from build123d import *

# Parameters (mm, degrees)
SKETCH1_W               = 20
SKETCH1_H               = 13
SKETCH1_R               = 1.2
BOSS_EXTRUDE1_DEPTH     = 5.8
SKETCH2_R               = 2.5
CUT_EXTRUDE1_DEPTH      = 2
SKETCH3_R               = 1.5
CUT_EXTRUDE2_DEPTH      = 10
FILLET1_R               = 10
FILLET2_R               = 5
FILLET3_R               = 2
FILLET4_R               = 1
SKETCH5_R               = 1.2
BOSS_EXTRUDE2_DEPTH     = 3.9
CUT_EXTRUDE3_DEPTH      = 26.750534103
CUT_EXTRUDE3_DEPTH_BACK = 26.750534103
SKETCH6_R               = 1


with BuildPart() as part:
    # Sketch1 → Boss-Extrude1 (new body)
    with BuildSketch(Plane.XY):
        with Locations((10, 6.5)):
            Rectangle(SKETCH1_W, SKETCH1_H)
        with Locations((16.5, 5)):
            Circle(SKETCH1_R, mode=Mode.SUBTRACT)
    extrude(amount=BOSS_EXTRUDE1_DEPTH)

    # Sketch2 → Cut-Extrude1 (cut)
    with BuildSketch(Plane.XY.offset(5.8)):
        with Locations((16.5, 5)):
            Circle(SKETCH2_R)
    extrude(amount=-CUT_EXTRUDE1_DEPTH, mode=Mode.SUBTRACT)

    # Sketch3 → Cut-Extrude2 (cut)
    with BuildSketch(Plane.ZY):
        with Locations((2.8, 5)):
            Circle(SKETCH3_R)
    extrude(amount=-CUT_EXTRUDE2_DEPTH, mode=Mode.SUBTRACT)

    # Fillet1
    fillet1_edges = [part.edges().sort_by_distance(p)[0] for p in [
        (20, 13, 2.9),
    ]]
    fillet(fillet1_edges, radius=FILLET1_R)

    # Fillet2
    fillet2_edges = [part.edges().sort_by_distance(p)[0] for p in [
        (0, 13, 2.9),
    ]]
    fillet(fillet2_edges, radius=FILLET2_R)

    # Fillet3
    fillet3_edges = [part.edges().sort_by_distance(p)[0] for p in [
        (0, 0, 2.9),
        (20, 0, 2.9),
    ]]
    fillet(fillet3_edges, radius=FILLET3_R)

    # Fillet4
    # the kernel refuses this fillet: 1 mm, written as the material it takes off along each edge
    with BuildSketch(Plane(origin=(5, 13, 5.8), x_dir=(0, 0, -1), z_dir=(1, 0, 0))) as fillet4_piece_1:
        with BuildLine():
            CenterArc((FILLET4_R, -FILLET4_R), FILLET4_R, 90, 90)
            Line((0, -FILLET4_R), (0, 0))
            Line((0, 0), (FILLET4_R, 0))
        make_face()
    extrude(amount=5, mode=Mode.SUBTRACT)
    with BuildSketch(Plane(origin=(10, 3, 5.8), x_dir=(0, 1, 0), z_dir=(-1, 0, 0))) as fillet4_piece_2:
        with BuildLine():
            CenterArc((10 - FILLET4_R, FILLET4_R), FILLET4_R, 270, 90)
            Line((10 - FILLET4_R, 0), (10, 0))
            Line((10, 0), (10, FILLET4_R))
        make_face()
    revolve(axis=Axis((10, 3, 5.8), (0, 0, -1)), revolution_arc=90, mode=Mode.SUBTRACT)
    with BuildSketch(Plane(origin=(0, 2, 5.8), x_dir=(0, 0, -1), z_dir=(0, 1, 0))) as fillet4_piece_3:
        with BuildLine():
            CenterArc((FILLET4_R, -FILLET4_R), FILLET4_R, 90, 90)
            Line((0, -FILLET4_R), (0, 0))
            Line((0, 0), (FILLET4_R, 0))
        make_face()
    extrude(amount=6, mode=Mode.SUBTRACT)
    with BuildSketch(Plane(origin=(5, 8, 5.8), x_dir=(0, 1, 0), z_dir=(1, 0, 0))) as fillet4_piece_4:
        with BuildLine():
            CenterArc((5 - FILLET4_R, -FILLET4_R), FILLET4_R, 0, 90)
            Line((5 - FILLET4_R, 0), (5, 0))
            Line((5, 0), (5, -FILLET4_R))
        make_face()
    revolve(axis=Axis((5, 8, 5.8), (0, 0, 1)), revolution_arc=90, mode=Mode.SUBTRACT)
    with BuildSketch(Plane(origin=(20, 3, 5.8), x_dir=(0, 0, -1), z_dir=(0, -1, 0))) as fillet4_piece_5:
        with BuildLine():
            CenterArc((FILLET4_R, -FILLET4_R), FILLET4_R, 90, 90)
            Line((0, -FILLET4_R), (0, 0))
            Line((0, 0), (FILLET4_R, 0))
        make_face()
    extrude(amount=1, mode=Mode.SUBTRACT)
    with BuildSketch(Plane(origin=(18, 0, 5.8), x_dir=(0, 0, -1), z_dir=(-1, 0, 0))) as fillet4_piece_6:
        with BuildLine():
            CenterArc((FILLET4_R, -FILLET4_R), FILLET4_R, 90, 90)
            Line((0, -FILLET4_R), (0, 0))
            Line((0, 0), (FILLET4_R, 0))
        make_face()
    extrude(amount=16, mode=Mode.SUBTRACT)
    with BuildSketch(Plane(origin=(2, 2, 5.8), x_dir=(-1, 0, 0), z_dir=(0, 1, 0))) as fillet4_piece_7:
        with BuildLine():
            CenterArc((2 - FILLET4_R, -FILLET4_R), FILLET4_R, 0, 90)
            Line((2 - FILLET4_R, 0), (2, 0))
            Line((2, 0), (2, -FILLET4_R))
        make_face()
    revolve(axis=Axis((2, 2, 5.8), (0, 0, 1)), revolution_arc=90, mode=Mode.SUBTRACT)
    with BuildSketch(Plane(origin=(18, 2, 5.8), x_dir=(1, 0, 0), z_dir=(0, 1, 0))) as fillet4_piece_8:
        with BuildLine():
            CenterArc((2 - FILLET4_R, FILLET4_R), FILLET4_R, 270, 90)
            Line((2 - FILLET4_R, 0), (2, 0))
            Line((2, 0), (2, FILLET4_R))
        make_face()
    revolve(axis=Axis((18, 2, 5.8), (0, 0, -1)), revolution_arc=90, mode=Mode.SUBTRACT)

    # Sketch5 → Boss-Extrude2 (add)
    with BuildSketch(Plane(origin=(0, 0, 0), x_dir=(-1, 0, 0), z_dir=(0, 0, -1))):
        with BuildLine():
            Line((-20, 3), (-20, 2))
            ThreePointArc((-20, 2), (-19.414213562, 0.585786438), (-18, 0))
            Line((-18, 0), (-2, 0))
            ThreePointArc((-2, 0), (-0.585786438, 0.585786438), (0, 2))
            Line((0, 2), (0, 8))
            ThreePointArc((0, 8), (-1.464466094, 11.535533906), (-5, 13))
            Line((-5, 13), (-10, 13))
            ThreePointArc((-10, 13), (-17.071067812, 10.071067812), (-20, 3))
        make_face()
        with Locations((-16.5, 5)):
            Circle(SKETCH5_R, mode=Mode.SUBTRACT)
    extrude(amount=BOSS_EXTRUDE2_DEPTH)

    # Sketch6 → Cut-Extrude3 (cut, two sides: drawn at the far end of the back side and taken through both)
    with BuildSketch(Plane.XY.offset(5.8).offset(-CUT_EXTRUDE3_DEPTH_BACK)):
        with Locations((10.515506471, 9.481609927)):
            Circle(SKETCH6_R)
    extrude(amount=CUT_EXTRUDE3_DEPTH + CUT_EXTRUDE3_DEPTH_BACK, mode=Mode.SUBTRACT)


solid = part.part
Part model, mm, in its own coordinate system. A direction names the side the tool comes from. Round coordinates to 2 decimals unless told otherwise and drop trailing zeros. Write each loop counter-clockwise with the first axis right and the second up, starting at its lowest first coordinate (ties: lowest second). Pieces come first, ordered by that corner, then holes. Notation, with made-up numbers: (-14.5, 57) - (1.5, 57) arc R16 ccw to (1.5, 63) - close; hole circle Ø10 at (-12, -16). An arc over 180 degrees is marked (long way). Use CSV: the item, a comma, the result in double quotes.
Item 1: Wall check: L1, parallel to Y at x = 8, z = 2.8; L2, parallel to Z at x = 14.25, y = 11; L3, parallel to Y at x = 6.75, z = 1.75. Give the ranges that are in metal, low to high.
Results list:
L1,"y = 0 to 3.5, 6.5 to 13"
L2,"z = -3.9 to 5.8"
L3,"y = 0 to 3.93, 6.07 to 13"
Item 2: Flat gauge pins, fed straight in: P1, Ø1.8, axis at y = 5, z = 2.8, coming from the -X side; P2, Ø1.4, axis at x = 16.5, y = 5, coming from the +Z side; P3, Ø4, axis at x = 17.5, z = -2, coming from the +Y side. Where does each tip first touch, or does it go through?
Results list:
P1,"stops at x = 10"
P2,"passes through"
P3,"stops at y = 11.35"
Item 3: Pull direction Y, two halves, no side cores. Call faces 4 (the flat face through (18, 6, 3.8)), 5 (the cylindrical face through (19.43, 0.6, 0.51)), 6 (the cylindrical face through (7.465, 12.715, 5.499)), 7 (the flat face through (10, 7, -3.9)): pulls with the +Y half, pulls with the -Y half, needs draft (parallel to the pull), parting line crosses it, or undercut.
Results list:
face 4,"undercut"
face 5,"pulls with the -Y half"
face 6,"pulls with the +Y half"
face 7,"needs draft"
Item 4: Slice it at B-B, the plane z = 2.8. Write the cut outline in (x, y).
Results list:
outline,"(0, 2) arc R2 ccw to (2, 0) - (18, 0) arc R2 ccw to (20, 2) - (20, 3) arc R10 ccw to (10, 13) - (5, 13) arc R5 ccw to (0, 8) - (0, 6.5) - (10, 6.5) - (10, 3.5) - (0, 3.5) - close; hole circle Ø2 at (10.52, 9.48); hole circle Ø2.4 at (16.5, 5)"
Item 5: Slice it at A-A, the plane z = -2. Write the cut outline in (x, y).
Results list:
outline,"(0, 2) arc R2 ccw to (2, 0) - (18, 0) arc R2 ccw to (20, 2) - (20, 3) arc R10 ccw to (10, 13) - (5, 13) arc R5 ccw to (0, 8) - close; hole circle Ø2 at (10.52, 9.48); hole circle Ø2.4 at (16.5, 5)"
Item 6: Tool access for faces 1 (the cylindrical face through (19.715, 2.507, 5.499)), 2 (the cylindrical face through (14, 5, 5)), 3 (the flat face through (10, 5, 3)): list every direction of +Z, -Z, +X, -X, +Y, -Y with a clear straight run to the whole face (end or side of a thin tool).
Results list:
face 1,"+Z, +X, +Y, -Y"
face 2,"+Z"
face 3,"-X"
